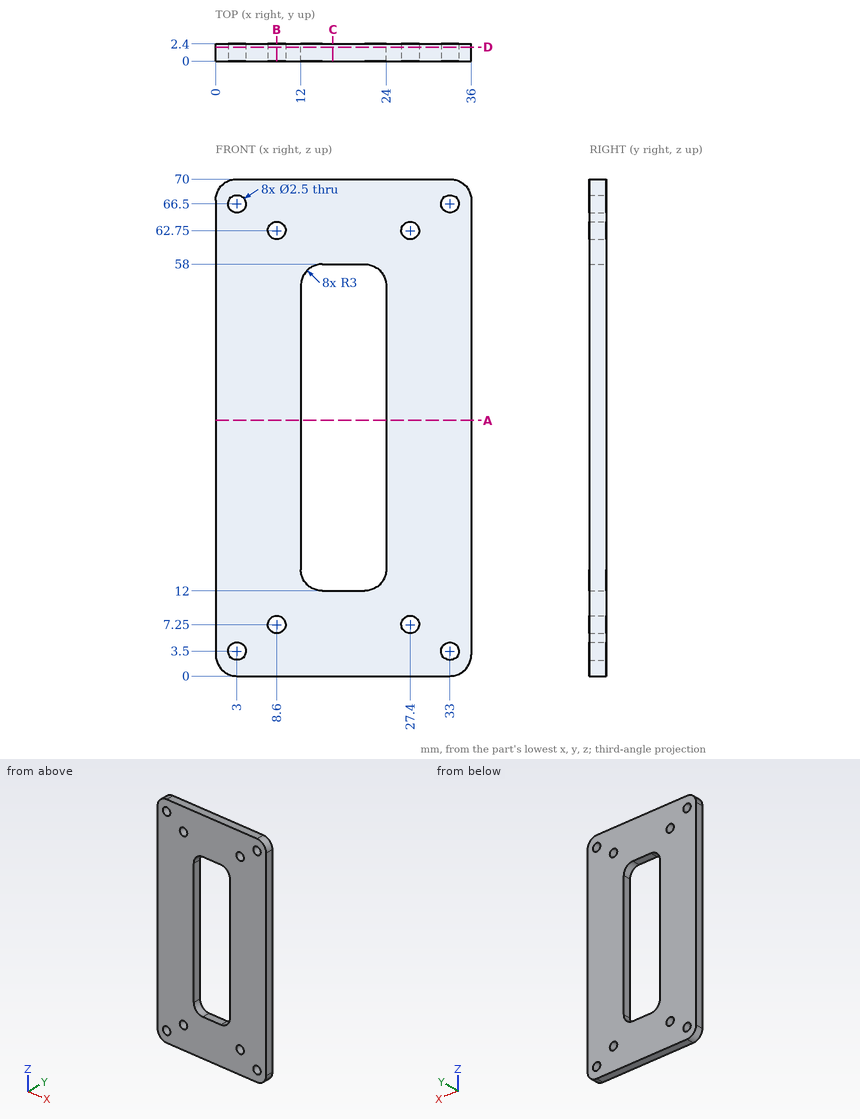
Job drawing, mm, ordinate dimensions from the low corner. One solid piece. Coordinates: 2 decimals unless noted, no trailing zeros. Write each loop counter-clockwise with the first axis right and the second up, starting at its lowest first coordinate (ties: lowest second). Pieces come first, ordered by that corner, then holes. Notation, with made-up numbers: M -34,82.5 L -29,82.5 A36 cw -29,118.5 Z; hole C 31,-28.75 d11. An arc over 180 degrees is marked long. Answer as a JSON object with one key per item and string values. Group by question number.
1) Saw through at C-C (x = 16.5). Write the cut outline in (y, z).
2) Saw through at B-B (x = 8.6). Write the cut outline in (y, z), plus the area to 3 significant figures.
3) Saw through at A-A (z = 36). Write the cut outline in (x, y).
4) Pin check, flat tips, straight feed: pin 1 Ø2 at (x, z) = (8.6, 62.75) entering from -Y; pin 2 Ø12 at (x, z) = (15, 45.5) entering from +Y. Stop position of each tip, or through.
5) Wall check: line 1 (Z direction, x = 33, y = 1.2); line 2 (X direction, y = 0.5, z = 62.75); line 3 (X direction, y = 1.5, z = 66.5). Give the ranges that are in metal, low to high. Write a range as from..to.
6) Saw through at D-D (y = 1.95). Give the number of separate pieces and of enclosed holes in the cut face, plus the area to 3 significant figures.
Values follow:
{
 "1": {"outline": "M 0,0 L 2.4,0 L 2.4,12 L 0,12 Z; M 0,58 L 2.4,58 L 2.4,70 L 0,70 Z"},
 "2": {"outline": "M 0,0 L 2.4,0 L 2.4,6 L 0,6 Z; M 0,8.5 L 2.4,8.5 L 2.4,61.5 L 0,61.5 Z; M 0,64 L 2.4,64 L 2.4,70 L 0,70 Z", "area": "156 mm2"},
 "3": {"outline": "M 0,0 L 12,0 L 12,2.4 L 0,2.4 Z; M 24,0 L 36,0 L 36,2.4 L 24,2.4 Z"},
 "4": {"pin 1": "passes through", "pin 2": "stops at y = 2.4"},
 "5": {"line 1": "z = 0..2.25, 4.75..65.25, 67.75..70", "line 2": "x = 0..7.35, 9.85..26.15, 28.65..36", "line 3": "x = 0..1.75, 4.25..31.75, 34.25..36"},
 "6": {"separate pieces": "1", "enclosed holes": "9", "area": "1,930 mm2"}
}
